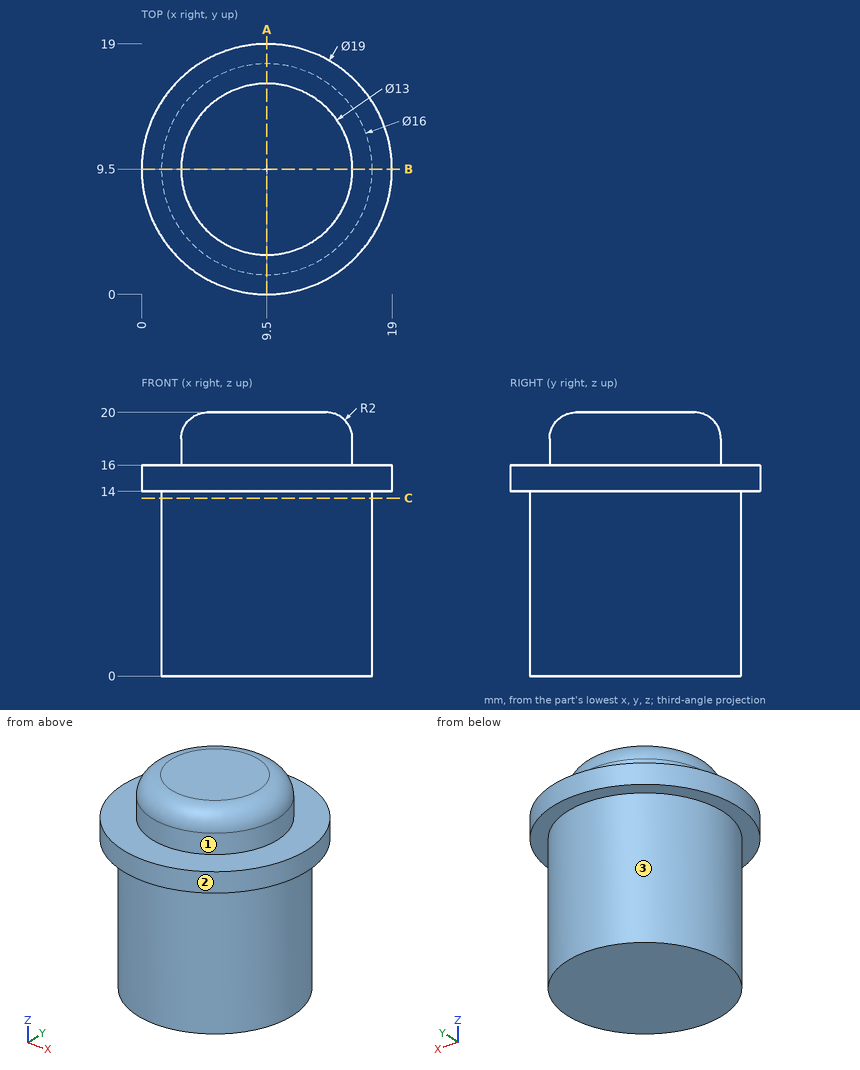
Source: three-view drawing plus pictorial views. Frame: mm from the lowest corner of the part. A direction names the side the tool comes from. Coordinates: 2 decimals unless noted, no trailing zeros. Order: outer loops, then holes, each group sorted by start corner. A loop starts at its lowest first (then second) coordinate and runs counter-clockwise, first axis right, second up.
Item 1: Set-up query: the marked faces 1, 2 and 3. Return all of +Z, -Z, +X, -X, +Y, -Y with unobstructed straight access to the full face (end or side cutting, diameter ignored); none if empty.
Output values:
face 1: +Z
face 2: +Z, -Z
face 3: -Z
Item 2: Material intervals for line 1 (Z direction, x = 6.75, y = 13.25); line 2 (Z direction, x = 3.75, y = 2.5); line 3 (Y direction, x = 9.5, z = 13), sorted ascending.
Output values:
line 1: z = 0 to 19.99
line 2: z = 14 to 16
line 3: y = 1.5 to 17.5
Item 3: Cut plane A-A (x = 9.5). Return loops of the section in (y, z), plus the area to 3 significant figures.
Output values:
outline: (0, 14) - (1.5, 14) - (1.5, 0) - (17.5, 0) - (17.5, 14) - (19, 14) - (19, 16) - (16, 16) - (16, 18) arc R2 ccw to (14, 20) - (5, 20) arc R2 ccw to (3, 18) - (3, 16) - (0, 16) - close
area: 312 mm2
Item 4: First-contact query: P1, Ø3, axis at x = 4, z = 3, coming from the -Y side; P2, Ø1, axis at y = 4.5, z = 10, coming from the +X side; P3, Ø4, axis at y = 15, z = 4, coming from the +X side. Flat tips, straight axial feed; report the tip coordinate or a pass-through.
Output values:
P1: stops at y = 2.57
P2: stops at x = 16.11
P3: stops at x = 16.69
Item 5: Cut plane C-C (z = 13.5). Return loops of the section in (x, y).
Output values:
outline: circle Ø16 at (9.5, 9.5)
